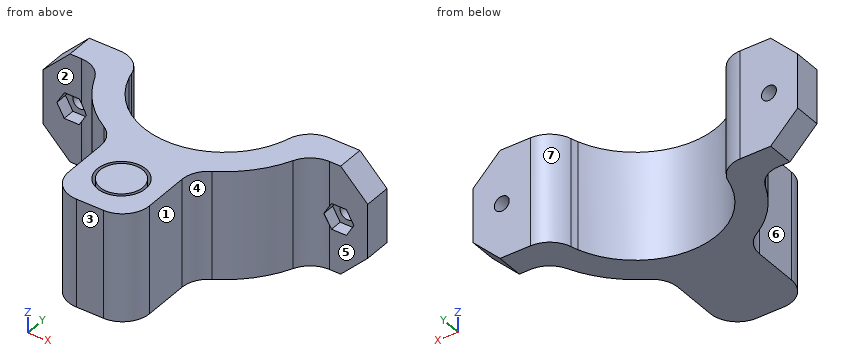
```python
from build123d import *

# Parameters (mm, degrees)
F1_DEPTH     = 50.8
F3_DEPTH     = 12.7
F4_SIZE      = 12.7
F5_R         = 11.35
F5_R_2       = 10
F6_DEPTH     = 44.45
F7_T1_DEPTH  = 50.8
F7_T6_DEPTH  = 73.3295570728
F7_T11_DEPTH = 73.3295570728
F7_T16_DEPTH = 73.3295570728
F7_T21_DEPTH = 73.3295570728
F7_T23_DEPTH = 114.3
F8_R         = 3.5
F9_DEPTH     = 50.801
F10_W        = 183.8439181447
F10_H        = 157.3934331536
F11_DEPTH    = 63.5
F12_R        = 12.7
F13_R        = 3.5
F13_W        = 17.6573731005
F13_H        = 18.0775066838
F14_DEPTH    = 7


# Not quite as in the source:
# - a fillet or chamfer that OpenCascade refuses, or shapes differently, is made with other operations: its cross-section is extruded or revolved along the edge and cut away or added


with BuildPart() as f1:
    # F0 (on Top) → F1 (new body)
    with BuildSketch(Plane.XY):
        with BuildLine():
            ThreePointArc((-35.9210244843, 12.7), (0, 38.1), (35.9210244843, 12.7))
            Line((35.9210244843, 12.7), (49.1868884968, 12.7))
            ThreePointArc((49.1868884968, 12.7), (0, 50.8), (-49.1868884968, 12.7))
            Line((-49.1868884968, 12.7), (-35.9210244843, 12.7))
        make_face()
        with BuildLine():
            ThreePointArc((-49.1868884968, -12.7), (-50.8, 0), (-49.1868884968, 12.7))
            Line((-49.1868884968, 12.7), (-76.2, 12.7))
            Line((-76.2, 12.7), (-76.2, -12.7))
            Line((-76.2, -12.7), (-49.1868884968, -12.7))
        make_face()
        with BuildLine():
            ThreePointArc((-35.9210244843, -12.7), (-38.1, 0), (-35.9210244843, 12.7))
            Line((-35.9210244843, 12.7), (-49.1868884968, 12.7))
            ThreePointArc((-49.1868884968, 12.7), (-50.8, 0), (-49.1868884968, -12.7))
            Line((-49.1868884968, -12.7), (-35.9210244843, -12.7))
        make_face()
        with BuildLine():
            ThreePointArc((35.9210244843, 12.7), (37.5513051228, 6.4427853895), (38.1, 0))
            ThreePointArc((38.1, 0), (37.5513051228, -6.4427853895), (35.9210244843, -12.7))
            Line((35.9210244843, -12.7), (49.1868884968, -12.7))
            ThreePointArc((49.1868884968, -12.7), (50.3951085704, -6.4010180581), (50.8, 0))
            ThreePointArc((50.8, 0), (50.3951085704, 6.4010180581), (49.1868884968, 12.7))
            Line((49.1868884968, 12.7), (35.9210244843, 12.7))
        make_face()
        with BuildLine():
            Line((76.2, 12.7), (49.1868884968, 12.7))
            ThreePointArc((49.1868884968, 12.7), (50.3951085704, 6.4010180581), (50.8, 0))
            ThreePointArc((50.8, 0), (50.3951085704, -6.4010180581), (49.1868884968, -12.7))
            Line((49.1868884968, -12.7), (76.2, -12.7))
            Line((76.2, -12.7), (76.2, 12.7))
        make_face()
        with BuildLine():
            ThreePointArc((-19.05, -32.9955678842), (-29.2989914869, -24.3552683798), (-35.9210244843, -12.7))
            Line((-35.9210244843, -12.7), (-49.1868884968, -12.7))
            ThreePointArc((-49.1868884968, -12.7), (-38.2071387235, -33.479165918), (-19.05, -47.0928603931))
            Line((-19.05, -47.0928603931), (-19.05, -32.9955678842))
        make_face()
        with BuildLine():
            Line((49.1868884968, -12.7), (35.9210244843, -12.7))
            ThreePointArc((35.9210244843, -12.7), (29.2989914869, -24.3552683798), (19.05, -32.9955678842))
            Line((19.05, -32.9955678842), (19.05, -47.0928603931))
            ThreePointArc((19.05, -47.0928603931), (38.2071387235, -33.479165918), (49.1868884968, -12.7))
        make_face()
        with BuildLine():
            Line((19.05, -47.0928603931), (19.05, -32.9955678842))
            ThreePointArc((19.05, -32.9955678842), (0, -38.1), (-19.05, -32.9955678842))
            Line((-19.05, -32.9955678842), (-19.05, -47.0928603931))
            ThreePointArc((-19.05, -47.0928603931), (0, -50.8), (19.05, -47.0928603931))
        make_face()
        with BuildLine():
            Line((19.05, -88.9), (19.05, -47.0928603931))
            ThreePointArc((19.05, -47.0928603931), (0, -50.8), (-19.05, -47.0928603931))
            Line((-19.05, -47.0928603931), (-19.05, -88.9))
            Line((-19.05, -88.9), (19.05, -88.9))
        make_face()
    extrude(amount=F1_DEPTH)

    # F2 (on face) → F3 (cut)
    with BuildSketch(Plane.XZ.offset(12.7)):
        Polygon((-55.6935602012, 25.3597094836), (-59.1586096141, 31.4419321502), (-66.1584936613, 31.4822226666), (-69.6933282956, 25.4402905164), (-66.2282788827, 19.3580678498), (-59.2283948355, 19.3177773334), align=None)
        Polygon((59.1938884968, 31.4621778265), (55.6938884968, 25.4), (59.1938884968, 19.3378221735), (66.1938884968, 19.3378221735), (69.6938884968, 25.4), (66.1938884968, 31.4621778265), align=None)
    extrude(amount=-F3_DEPTH, mode=Mode.SUBTRACT)

    # F4
    f4_edges = [f1.edges().sort_by_distance(p)[0] for p in [
        (-76.2, 0, 50.8),
        (-76.2, 0, 0),
        (76.2, 0, 50.8),
        (76.2, 0, 0),
    ]]
    chamfer(f4_edges, length=F4_SIZE)

    # F5 (on face) → F6 (cut)
    with BuildSketch(Plane.XY.offset(50.8)):
        with Locations((0, -67.9964301965)):
            Circle(F5_R)
        with Locations((0, -67.9964301965)):
            Circle(F5_R_2, mode=Mode.SUBTRACT)
    extrude(amount=-F6_DEPTH, mode=Mode.SUBTRACT)

    # F7: fillet of radius 12.7 on 8 edges, made by hand

    # F7_s2 → F7_t1 (join)
    with BuildSketch(Plane.XY):
        with BuildLine():
            ThreePointArc((-25.4, -43.9940905122), (-20.7514773719, -48.6426131403), (-19.05, -54.9926131403))
            Line((-19.05, -54.9926131403), (-19.05, -47.0928603931))
            ThreePointArc((-19.05, -47.0928603931), (-22.2789411484, -45.6540116672), (-25.4, -43.9940905122))
        make_face()
        with BuildLine():
            ThreePointArc((25.4, -43.9940905122), (20.7514773719, -48.6426131403), (19.05, -54.9926131403))
            Line((19.05, -54.9926131403), (19.05, -47.0928603931))
            ThreePointArc((19.05, -47.0928603931), (22.2789411484, -45.6540116672), (25.4, -43.9940905122))
        make_face()
    extrude(amount=F7_T1_DEPTH)


with BuildPart() as f7_tool4:
    # F7_s5 → F7_t6 (new body)
    with BuildSketch(Plane.XY):
        with BuildLine():
            ThreePointArc((58.1987113259, -12.7), (51.2426348456, -14.774417663), (46.5589690608, -20.32))
            ThreePointArc((46.5589690608, -20.32), (48.0243002017, -16.562203662), (49.1868884968, -12.7))
            Line((49.1868884968, -12.7), (58.1987113259, -12.7))
        make_face()
    extrude(amount=F7_T6_DEPTH)

    split(bisect_by=Plane(origin=(52.7689390007, 0, 30.4661611369), x_dir=(0, 1, 0), z_dir=(-0.8660254038, 0, -0.5)), keep=Keep.TOP)


with BuildPart() as f1_1:
    add(f1.part)

    # F7_t3: union F7_tool4
    add(f7_tool4.part)


with BuildPart() as f7_tool9:
    # F7_s10 → F7_t11 (new body)
    with BuildSketch(Plane.XY.offset(-22.5295570728)):
        with BuildLine():
            ThreePointArc((58.1987113259, -12.7), (51.2426348456, -14.774417663), (46.5589690608, -20.32))
            ThreePointArc((46.5589690608, -20.32), (48.0243002017, -16.562203662), (49.1868884968, -12.7))
            Line((49.1868884968, -12.7), (58.1987113259, -12.7))
        make_face()
    extrude(amount=F7_T11_DEPTH)

    split(bisect_by=Plane(origin=(30.7718937446, 0, -17.7661611369), x_dir=(0, 1, 0), z_dir=(-0.8660254038, 0, 0.5)), keep=Keep.TOP)


with BuildPart() as f1_2:
    add(f1_1.part)

    # F7_t8: union F7_tool9
    add(f7_tool9.part)


with BuildPart() as f7_tool14:
    # F7_s15 → F7_t16 (new body)
    with BuildSketch(Plane.XY):
        with BuildLine():
            ThreePointArc((-58.1987113259, -12.7), (-51.2426348456, -14.774417663), (-46.5589690608, -20.32))
            ThreePointArc((-46.5589690608, -20.32), (-48.0243002017, -16.562203662), (-49.1868884968, -12.7))
            Line((-49.1868884968, -12.7), (-58.1987113259, -12.7))
        make_face()
    extrude(amount=F7_T16_DEPTH)

    split(bisect_by=Plane(origin=(-52.5449689068, 0, 30.7414534512), x_dir=(0, 1, 0), z_dir=(0.8631331643, 0, -0.5049763763)), keep=Keep.TOP)


with BuildPart() as f1_3:
    add(f1_2.part)

    # F7_t13: union F7_tool14
    add(f7_tool14.part)


with BuildPart() as f7_tool19:
    # F7_s20 → F7_t21 (new body)
    with BuildSketch(Plane.XY.offset(-22.5295570728)):
        with BuildLine():
            ThreePointArc((-58.1987113259, -12.7), (-51.2426348456, -14.774417663), (-46.5589690608, -20.32))
            ThreePointArc((-46.5589690608, -20.32), (-48.0243002017, -16.562203662), (-49.1868884968, -12.7))
            Line((-49.1868884968, -12.7), (-58.1987113259, -12.7))
        make_face()
    extrude(amount=F7_T21_DEPTH)

    split(bisect_by=Plane(origin=(-31.1394890128, 0, -17.7402035465), x_dir=(0, 1, 0), z_dir=(0.8688889524, 0, 0.495007059)), keep=Keep.TOP)


with BuildPart() as f1_4:
    add(f1_3.part)

    # F7_t18: union F7_tool19
    add(f7_tool19.part)

    # F7_s24 → F7_t23 (cut)
    with BuildSketch(Plane.XY.offset(-31.75)):
        with BuildLine():
            ThreePointArc((-6.35, -88.9), (-15.3302561211, -85.1802561211), (-19.05, -76.2))
            Line((-19.05, -76.2), (-19.05, -88.9))
            Line((-19.05, -88.9), (-6.35, -88.9))
        make_face()
        with BuildLine():
            ThreePointArc((19.05, -76.2), (15.3302561211, -85.1802561211), (6.35, -88.9))
            Line((6.35, -88.9), (19.05, -88.9))
            Line((19.05, -88.9), (19.05, -76.2))
        make_face()
    extrude(amount=F7_T23_DEPTH, mode=Mode.SUBTRACT)

    # F8 (on face) → F9 (cut, through all)
    with BuildSketch(Plane.XZ):
        with Locations((-62.6585516377, 25.4402905164)):
            Circle(F8_R)
        with Locations((62.6938884968, 25.4402905164)):
            Circle(F8_R)
    extrude(amount=-F9_DEPTH, mode=Mode.SUBTRACT)

    # F10 (on Front) → F11 (cut)
    with BuildSketch(Plane.XZ):
        with Locations((-6.0164444149, -2.5229565799)):
            Rectangle(F10_W, F10_H)
    extrude(amount=-F11_DEPTH, mode=Mode.SUBTRACT)

    # F12
    f12_edges = [f1_4.edges().sort_by_distance(p)[0] for p in [
        (38.1, 0, 25.4),
        (-38.1, 0, 25.4),
    ]]
    fillet(f12_edges, radius=F12_R)

    # F13 (on face) → F14 (join)
    with BuildSketch(Plane(origin=(0, 0, 0), x_dir=(-1, 0, 0), z_dir=(0, 1, 0))):
        Polygon((-55.6938884968, 25.4), (-59.1938884968, 31.4621778265), (-66.1938884968, 31.4621778265), (-69.6938884968, 25.4), (-66.1938884968, 19.3378221735), (-59.1938884968, 19.3378221735), align=None)
        with Locations((-62.6938884968, 25.4)):
            Circle(F13_R, mode=Mode.SUBTRACT)
        with Locations((63.3883532137, 24.6192668565)):
            Rectangle(F13_W, F13_H)
        with Locations((62.6936761559, 25.3597094836)):
            Circle(F13_R, mode=Mode.SUBTRACT)
    extrude(amount=-F14_DEPTH)


solid = f1_4.part
```
Here's how the part is built. I have some questions about the finished solid (model axes, mm). Face numbers are marked on the shaded views. A direction names the side the tool comes from. Give positions to 0.01 mm unless a question says otherwise; leave off trailing zeros. Write each loop counter-clockwise with the first axis right and the second up, starting at its lowest first coordinate (ties: lowest second). Pieces come first, ordered by that corner, then holes. Notation, with made-up numbers: M 41.25,-1 L 77.25,-1 A17 cw 77.25,8 Z; hole C 44.25,-0.5 d8. An arc over 180 degrees is marked long. Put each result on its own line as item: value. Start each with the question number.
Item 1: If we section it at A-A, the plane z = 17: Write out the boundary of the cut face in (x, y) (3 decimals).
Item 2: If we section it at D-D, the plane x = -61: Write out the boundary of the cut face in (y, z), then the cut area to 3 significant figures.
Item 3: If we section it at C-C, the plane y = -30.5: Write out the boundary of the cut face in (x, z) (3 decimals), then the cut area to 3 significant figures.
Item 4: I need wall thicknesses on L1, parallel to Y at x = 0, z = 24; L2, parallel to Y at x = -0.5, z = 24; L3, parallel to X at y = -4, z = 25. Which ranges of each line are inside material? Lowest first, please. Write a range as from..to.
Item 5: Thinking about a two-plate mould opening in X: for the marked faces 4, 5, 6 and 7, which applies, +X half, -X half, draft (parallel to the pull), parting line (faces both ways), or undercut?
Item 6: Will these pins go through, and if not, where does the flat tip stop? pin 1 (9 mm diameter, centred on x = 69.5, z = 30, fed in from -Y); pin 2 (13.5 mm diameter, centred on x = 62.5, z = 27, fed in from -Y); pin 3 (23.5 mm diameter, centred on y = -70.5, z = 17.5, fed in from +X); pin 4 (3.5 mm diameter, centred on x = -64, z = 24.5, fed in from -Y).
Item 7: On a 3-axis mill with a long thin cutter (end or side, diameter ignored), from which of +Z, -Z, +X, -X, +Y, -Y can I reach the whole of each face in a straight line? I mean the marked faces 1, 2 and 3. Say none if no direction works.
Item 8: If we section it at B-B, the plane x = 0: Write out the boundary of the cut face in (y, z).
Values:
1. outline: M -76.2,-12.7 L -58.199,-12.7 A12.7 cw -46.559,-20.32 A50.8 ccw -25.4,-43.994 A12.7 cw -19.05,-54.993 L -19.05,-76.2 A12.7 ccw -6.35,-88.9 L 6.35,-88.9 A12.7 ccw 19.05,-76.2 L 19.05,-54.993 A12.7 cw 25.4,-43.994 A50.8 ccw 46.559,-20.32 A12.7 cw 58.199,-12.7 L 76.2,-12.7 L 76.2,0 L 49.187,0 A12.7 ccw 36.89,-9.525 A38.1 cw -36.89,-9.525 A12.7 ccw -49.187,0 L -76.2,0 Z; C 0,-67.996 d20; hole C 0,-67.996 d22.7
2. outline: M -12.7,0 L 0,0 L 0,22.3 L -7,22.3 L -7,19.33 L -12.7,19.33 Z; M -12.7,31.45 L -7,31.45 L -7,28.42 L 0,28.42 L 0,50.8 L -12.7,50.8 Z
2. area: 533 mm²
3. outline: M -40.625,0 L -22.833,0 L -22.833,50.8 L -40.625,50.8 Z; M 22.833,0 L 40.625,0 L 40.625,50.8 L 22.833,50.8 Z
3. area: 1,810 mm²
4. L1: -88.9..-79.35, -78..-58, -56.65..-38.1
4. L2: -88.9..-79.34, -77.98..-58.01, -56.66..-38.1
4. L3: -76.2..-66.18, -59.21..-39.93, 39.93..59.22, 66.17..76.2
5. face 4: +X half
5. face 5: draft
5. face 6: -X half
5. face 7: undercut
6. pin 1: y = -12.7
6. pin 2: y = -12.94
6. pin 3: x = 19.05
6. pin 4: through
7. face 1: +Z, -Z, +X, -Y
7. face 2: +Z, -Z, -X, -Y
7. face 3: +Z, -Z, +X, -X, -Y
8. outline: M -88.9,0 L -38.1,0 L -38.1,50.8 L -56.65,50.8 L -56.65,6.35 L -58,6.35 L -58,50.8 L -78,50.8 L -78,6.35 L -79.35,6.35 L -79.35,50.8 L -88.9,50.8 Z
